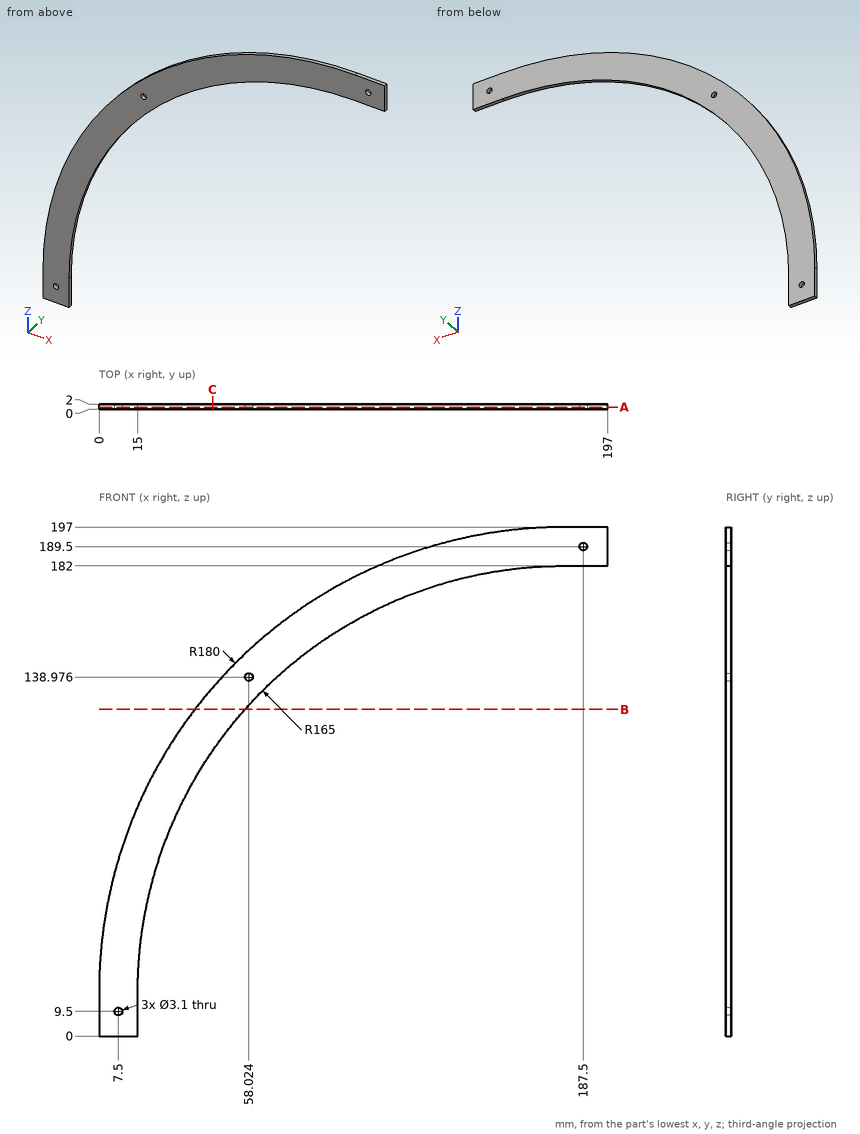
Could you check a few things on this drawing? It's one solid part, dimensions in mm from its lowest x, y, z. Coordinates: 2 decimals unless noted, no trailing zeros. Order: outer loops, then holes, each group sorted by start corner. A loop starts at its lowest first (then second) coordinate and runs counter-clockwise, first axis right, second up.
1. I need wall thicknesses on line 1 (Z direction, x = 187.5, y = 0.5); line 2 (X direction, y = 0.25, z = 10.5); line 3 (Z direction, x = 185.5, y = 0.9). Which ranges of each line are inside material? Lowest first, please.
2. If we section it at B-B (z = 126.5): Please give me the cut outline in (x, y), then the cut area to 3 significant figures.
3. If we section it at C-C (x = 44): Please give me the cut outline in (y, z).
4. If we section it at A-A (y = 0.8): Please give me the cut outline in (x, z).
5. I'm going to push flat-ended pins straight in: pin 1 (0.6 mm diameter, centred on y = 1.5, z = 5, fed in from +X); pin 2 (3 mm diameter, centred on x = 187.5, z = 189.5, fed in from +Y); pin 3 (1 mm diameter, centred on x = 190.5, y = 1, fed in from -Z); pin 4 (3.5 mm diameter, centred on x = 7.5, z = 9.5, fed in from +Y). Where does each tip first touch, or does it pass through?
Entries:
1. line 1: z = 182 to 187.95, 191.05 to 197
1. line 2: x = 0 to 6.32, 8.68 to 15
1. line 3: z = 182 to 197
2. outline: (37.14, 0) - (56.57, 0) - (56.57, 2) - (37.14, 2) - close
2. area: 38.9 mm2
3. outline: (0, 110.43) - (2, 110.43) - (2, 134.92) - (0, 134.92) - close
4. outline: (0, 0) - (15, 0) - (15, 17) arc R165 cw to (180, 182) - (197, 182) - (197, 197) - (180, 197) arc R180 ccw to (0, 17) - close; hole circle Ø3.1 at (7.5, 9.5); hole circle Ø3.1 at (58.02, 138.98); hole circle Ø3.1 at (187.5, 189.5)
5. pin 1: stops at x = 15
5. pin 2: passes through
5. pin 3: stops at z = 182
5. pin 4: stops at y = 2
